Build history of the part. All positions in model axes, mm. Face numbers are marked on the shaded views. A direction names the side the tool comes from. Round coordinates to 2 decimals unless told otherwise and drop trailing zeros. Order: outer loops, then holes, each group sorted by start corner. A loop starts at its lowest first (then second) coordinate and runs counter-clockwise, first axis right, second up. Notation, with made-up numbers: (25.25, 53.5) -> (48.25, 53.5) arc R16 cw to (48.25, 79.5) -> close; hole circle Ø8 at (-30.5, -5.5). An arc over 180 degrees is marked (long way). Answer as a JSON object with one key per item and string values.
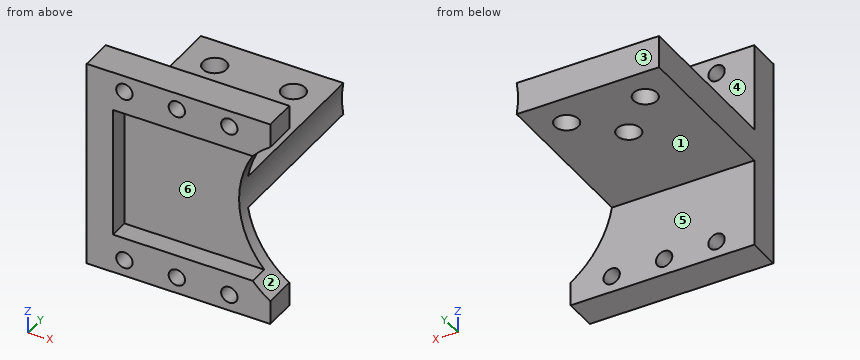
from build123d import *

# Parameters (mm, degrees)
SZKIC1_W                    = 20
SZKIC1_H                    = 20
DODANIE_WYCI_GNI_CIE1_DEPTH = 2
SZKIC3_R                    = 1.25
DODANIE_WYCI_GNI_CIE2_DEPTH = 5
SZKIC4_W                    = 24
SZKIC4_H                    = 5
DODANIE_WYCI_GNI_CIE3_DEPTH = 25
DODANIE_WYCI_GNI_CIE4_DEPTH = 4
SZKIC6_R                    = 15
WYTNIJ_WYCI_GNI_CIE1_DEPTH  = 34
OTW_R_POD_RUB_M31_D         = 3.6
OTW_R_POD_RUB_M31_DEPTH     = 24


with BuildPart() as part:
    # Szkic1 → Dodanie-wyciągnięcie1 (new body)
    with BuildSketch(Plane(origin=(0, 0, 0), x_dir=(1, 0, 0), z_dir=(0, 1, 0))):
        Rectangle(SZKIC1_W, SZKIC1_H)
    extrude(amount=DODANIE_WYCI_GNI_CIE1_DEPTH)

    # Szkic3 → Dodanie-wyciągnięcie2 (add)
    with BuildSketch(Plane(origin=(0, 2, 0), x_dir=(1, 0, 0), z_dir=(0, 1, 0))):
        Polygon((-14, 16), (-14, -16), (10, -16), (10, -10), (-10, -10), (-10, 10), (10, 10), (10, 16), align=None)
        with Locations(Location((-8.25, -13.5, 0), (0, 0, 270))):
            Circle(SZKIC3_R, mode=Mode.SUBTRACT)
        with Locations(Location((-0.25, -13.5, 0), (0, 0, 270))):
            Circle(SZKIC3_R, mode=Mode.SUBTRACT)
        with Locations(Location((7.75, -13.5, 0), (0, 0, 270))):
            Circle(SZKIC3_R, mode=Mode.SUBTRACT)
        with Locations(Location((-8.25, 13.5, 0), (0, 0, 270))):
            Circle(SZKIC3_R, mode=Mode.SUBTRACT)
        with Locations(Location((-0.25, 13.5, 0), (0, 0, 270))):
            Circle(SZKIC3_R, mode=Mode.SUBTRACT)
        with Locations(Location((7.75, 13.5, 0), (0, 0, 270))):
            Circle(SZKIC3_R, mode=Mode.SUBTRACT)
    extrude(amount=-DODANIE_WYCI_GNI_CIE2_DEPTH)

    # Szkic4 → Dodanie-wyciągnięcie3 (add)
    with BuildSketch(Plane(origin=(0, 2, 0), x_dir=(1, 0, 0), z_dir=(0, 1, 0))):
        with Locations((-2, 0)):
            Rectangle(SZKIC4_W, SZKIC4_H)
    extrude(amount=DODANIE_WYCI_GNI_CIE3_DEPTH)

    # Szkic5 → Dodanie-wyciągnięcie4 (add)
    with BuildSketch(Plane(origin=(10, 0, 0), x_dir=(0, 0, -1), z_dir=(1, 0, 0))):
        Polygon((-10, 0), (10, 0), (10, -3), (16, -3), (16, 2), (2.5, 2), (2.5, 27), (-2.5, 27), (-2.5, 2), (-16, 2), (-16, -3), (-10, -3), align=None)
    extrude(amount=DODANIE_WYCI_GNI_CIE4_DEPTH)

    # Szkic6 → Wytnij-wyciągnięcie1 (cut)
    with BuildSketch(Plane(origin=(0, 27, 0), x_dir=(1, 0, 0), z_dir=(0, 1, 0))):
        with Locations((22.5, 0)):
            Circle(SZKIC6_R)
    extrude(amount=-WYTNIJ_WYCI_GNI_CIE1_DEPTH, mode=Mode.SUBTRACT)

    # Otwór pod śrubę M31
    with Locations(Plane.XY.offset(2.5)):
        with Locations((3, 22), (-9, 22), (-3, 16)):
            Hole(OTW_R_POD_RUB_M31_D / 2, depth=OTW_R_POD_RUB_M31_DEPTH)


solid = part.part
1) Pull direction Z, two halves, no side cores. Call the marked faces 1, 2 and 3: pulls with the +Z half, pulls with the -Z half, needs draft (parallel to the pull), parting line crosses it, or undercut.
Checked values:
{"face 1": "pulls with the -Z half", "face 2": "undercut", "face 3": "needs draft"}
2) Probe L1, parallel to X at y = 0.6, z = -13.5; L2, parallel to X at y = -0.75, z = 0.5; L3, parallel to Z at x = -8, y = 15. List the from-to ranges inside material, lowest first. Write a range as from..to.
Checked values:
{"L1": "x = -14..-9.5, -7..-1.5, 1..6.5, 9..14", "L2": "x = -14..-10", "L3": "z = -2.5..2.5"}
3) Cut at B-B, the plane z = -13.5. Give the cut face in (x, y).
Checked values:
{"outline": "(-14, -3) -> (-9.5, -3) -> (-9.5, 2) -> (-14, 2) -> close; (-7, -3) -> (-1.5, -3) -> (-1.5, 2) -> (-7, 2) -> close; (1, -3) -> (6.5, -3) -> (6.5, 2) -> (1, 2) -> close; (9, -3) -> (14, -3) -> (14, 2) -> (9, 2) -> close"}
4) Which spindle directions (+Z, -Z, +X, -X, +Y, -Y) get a long thin tool onto all of the face, cutting with end or side? Do the marked faces 4, 5 and 6. Say none if no direction does.
Checked values:
{"face 4": "+Z, +X, -X, +Y", "face 5": "-Z, +X, -X, +Y", "face 6": "+X, -Y"}
5) Flat gauge pins, fed straight in: pin 1 Ø1.5 at (y, z) = (23, 1) entering from +X; pin 2 Ø4 at (x, y) = (-3, 16) entering from -Z; pin 3 Ø6.5 at (x, y) = (-7, 9.5) entering from +Z. Where does each tip first touch, or does it go through?
Checked values:
{"pin 1": "stops at x = 7.6", "pin 2": "stops at z = -2.5", "pin 3": "stops at z = 2.5"}
6) Cut at C-C, the plane x = 3. Give the cut face in (y, z).
Checked values:
{"outline": "(-3, -16) -> (2, -16) -> (2, -2.5) -> (20.2, -2.5) -> (20.2, 2.5) -> (2, 2.5) -> (2, 16) -> (-3, 16) -> (-3, 10) -> (0, 10) -> (0, -10) -> (-3, -10) -> close; (23.8, -2.5) -> (27, -2.5) -> (27, 2.5) -> (23.8, 2.5) -> close"}
7) Cut at A-A, the plane y = 16. Give the cut face in (x, z).
Checked values:
{"outline": "(-14, -2.5) -> (-4.8, -2.5) -> (-4.8, 2.5) -> (-14, 2.5) -> close; (-1.2, -2.5) -> (7.71, -2.5) arc R15 cw to (7.71, 2.5) -> (-1.2, 2.5) -> close"}
8) Cut at D-D, the plane x = -9. Give the cut face in (y, z).
Checked values:
{"outline": "(-3, -16) -> (2, -16) -> (2, -14.5) -> (-3, -14.5) -> close; (-3, -12.5) -> (2, -12.5) -> (2, -2.5) -> (20.2, -2.5) -> (20.2, 2.5) -> (2, 2.5) -> (2, 12.5) -> (-3, 12.5) -> (-3, 10) -> (0, 10) -> (0, -10) -> (-3, -10) -> close; (-3, 14.5) -> (2, 14.5) -> (2, 16) -> (-3, 16) -> close; (23.8, -2.5) -> (27, -2.5) -> (27, 2.5) -> (23.8, 2.5) -> close"}
